Input: dimensioned drawing with shaded views. Units: mm. Origin: part minimum x, y, z. A direction names the side the tool comes from. Coordinates: 2 decimals unless noted, no trailing zeros. Loops run counter-clockwise (first coordinate to the right, second up) from the corner with the lowest first, then second, coordinate; pieces in that order, holes last.
Item 1: Section C-C on y = 242. Return loops of the section in (x, z).
Item 2: Contact query for a flat-ended pin moving along its axis: P1, Ø1.5, axis at x = 21, y = 170, coming from the +Z side. Output: stop coordinate, or through.
Item 3: Section B-B on x = 58.5. Return loops of the section in (y, z), and give its area (3 significant figures).
Item 4: Reachability of the marked faces 1 and 2 from +Z, -Z, +X, -X, +Y, -Y: full face, straight path, thin tool, end or side. Return the list, or none.
Item 5: Section A-A on z = 83. Return loops of the section in (x, y).
Item 6: Ray query, line 1 along Z through (x, y) = (51, 168); line 2 along X through (y, z) = (246, 138.5). Return the intervals inside material, ascending.
Item 7: Pull-direction query (X, two-part tool) for the marked faces 3, 4, 5 and 6; classes: released by +X, released by -X, zero draft, split by the parting line, or undercut.
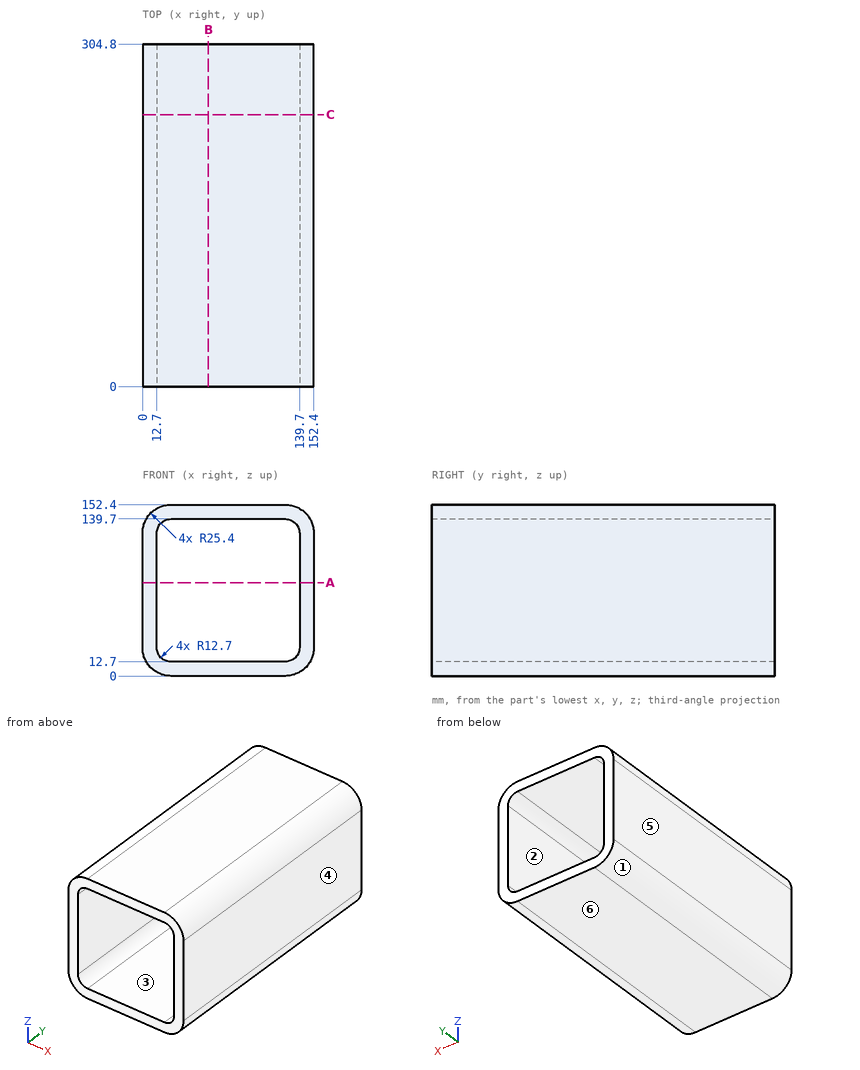
Results found:
1. outline: (0, 25.4) arc R25.4 ccw to (25.4, 0) - (127, 0) arc R25.4 ccw to (152.4, 25.4) - (152.4, 127) arc R25.4 ccw to (127, 152.4) - (25.4, 152.4) arc R25.4 ccw to (0, 127) - close; hole (12.7, 25.4) arc R12.7 ccw to (25.4, 12.7) - (127, 12.7) arc R12.7 ccw to (139.7, 25.4) - (139.7, 127) arc R12.7 ccw to (127, 139.7) - (25.4, 139.7) arc R12.7 ccw to (12.7, 127) - close
2. P1: stops at z = 152.14
3. outline: (0, 0) - (304.8, 0) - (304.8, 12.7) - (0, 12.7) - close; (0, 139.7) - (304.8, 139.7) - (304.8, 152.4) - (0, 152.4) - close
3. area: 7,740 mm2
4. face 1: -Z, -X, +Y, -Y
4. face 2: +Y, -Y
5. outline: (0, 0) - (12.7, 0) - (12.7, 304.8) - (0, 304.8) - close; (139.7, 0) - (152.4, 0) - (152.4, 304.8) - (139.7, 304.8) - close
6. line 1: z = 0 to 12.7, 139.7 to 152.4
6. line 2: x = 2.75 to 20.01, 132.39 to 149.65
7. face 3: undercut
7. face 4: released by +X
7. face 5: released by -X
7. face 6: zero draft
